Input: part model. Units: mm. Frame: model coordinates. Coordinates: 2 decimals unless noted, no trailing zeros. Order: outer loops, then holes, each group sorted by start corner. A loop starts at its lowest first (then second) coordinate and runs counter-clockwise, first axis right, second up. Notation, with made-up numbers: (62, 49.5) - (105, 49.5) arc R19 cw to (105, 75.5) - close; hole circle Ø10 at (-5.5, 38.25). An arc over 180 degrees is marked (long way). One line per question, with ' | ' between items. Start each with the question number.
Autodesk Inventor part; units mm, degrees
ref_plane "YZ Plane" through (0, 0, 0) normal (1, 0, 0) x (0, 1, 0)
ref_plane "XZ Plane" through (0, 0, 0) normal (0, 1, 0) x (-1, 0, 0)
ref_plane "XY Plane" through (0, 0, 0) normal (0, 0, 1) x (1, 0, 0)
sketch "Boceto1" plane through (0, 0, 0) normal (0, 1, 0) x (-1, 0, 0)
  arc A0 (120.2602, -12.5039) -> (120.7259, 12.475) centre (120.0354, -0.0059) ccw
  line L0 (2.2617, 19.3684) -> (120.7259, 12.475)
  line L1 (2.266, -19.3679) -> (119.9998, -12.5039)
  arc A1 (2.2617, 19.3684) -> (2.266, -19.3679) centre (0, 0) ccw
  circle A2 centre (120.0354, -0.0059) radius 1.5
  circle A3 centre (0, 0) radius 1.5
  circle A4 centre (0, -8) radius 1.5
  circle A5 centre (0, 8) radius 1.5
  line L2 (119.9998, -12.5039) -> (120.2602, -12.5039)
  dimension "d107" = 3
extrude "Extrusión1" add sketch "Boceto1" along normal blind 3
properties part number "planos robot"
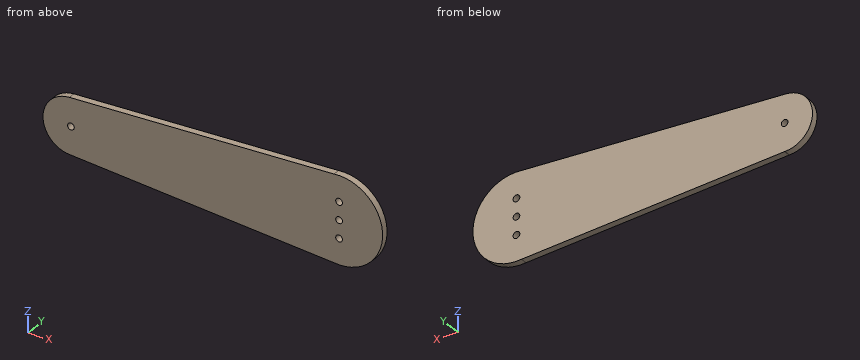
(1) Pin query (flat end, axial travel): pin 1 (1.5 mm diameter, centred on y = 1, z = -8, fed in from +X); pin 2 (1 mm diameter, centred on x = -104, y = 2, fed in from -Z); pin 3 (1.5 mm diameter, centred on y = 2.5, z = -5, fed in from -X). Return the tip coordinate at first contact, or that it passes through.
(2) Section B-B (z = -8). Output: boundary loops of the cut face in (x, y).
(3) Material intervals for line 1 along Z through (x, y) = (0, 1.45); line 2 along Z through (x, y) = (-6, 2.05); line 3 along X through (y, z) = (0.75, 7), sorted ascending. Write a range as from..to.
(4) Section A-A (x = 0). Output: boundary loops of the cut face in (y, z), then the cut area to 3 significant figures.
(5) Section C-C (y = 0.6). Output: boundary loops of the cut face in (x, z) (3 decimals).
(6) Section D-D (z = 8). Output: boundary loops of the cut face in (x, y).
Worked answers:
1) pin 1: stops at x = 18.1 | pin 2: stops at z = -13.47 | pin 3: stops at x = -131.79
2) outline: (-129.65, 0) - (-1.5, 0) - (-1.5, 3) - (-129.65, 3) - close; (1.5, 0) - (17.78, 0) - (17.78, 3) - (1.5, 3) - close
3) line 1: z = -19.5..-9.5, -6.5..-1.5, 1.5..6.5, 9.5..19.5 | line 2: z = -19.15..19.15 | line 3: x = -130.39..-1.12, 1.12..18.2
4) outline: (0, -19.5) - (3, -19.5) - (3, -9.5) - (0, -9.5) - close; (0, -6.5) - (3, -6.5) - (3, -1.5) - (0, -1.5) - close; (0, 1.5) - (3, 1.5) - (3, 6.5) - (0, 6.5) - close; (0, 9.5) - (3, 9.5) - (3, 19.5) - (0, 19.5) - close | area: 90.0 mm²
5) outline: (-120.726, 12.475) arc R12.5 ccw to (-120.26, -12.504) - (-120, -12.504) - (-2.266, -19.368) arc R19.5 ccw (long way) to (-2.262, 19.368) - close; hole circle Ø3 at (-120.035, -0.006); hole circle Ø3 at (0, -8); hole circle Ø3 at (0, 0); hole circle Ø3 at (0, 8)
6) outline: (-129.64, 0) - (-1.5, 0) - (-1.5, 3) - (-129.64, 3) - close; (1.5, 0) - (17.78, 0) - (17.78, 3) - (1.5, 3) - close
